Job drawing, mm, ordinate dimensions from the low corner. One solid piece. A direction names the side the tool comes from. Round coordinates to 2 decimals unless told otherwise and drop trailing zeros. Order: outer loops, then holes, each group sorted by start corner. A loop starts at its lowest first (then second) coordinate and runs counter-clockwise, first axis right, second up. Notation, with made-up numbers: (6.5, 57) -> (45.5, 57) arc R8 ccw to (45.5, 63) -> close; hole circle Ø8 at (40, -4.5). An arc over 180 degrees is marked (long way). Use CSV: the item, a comma, the result in double quotes.
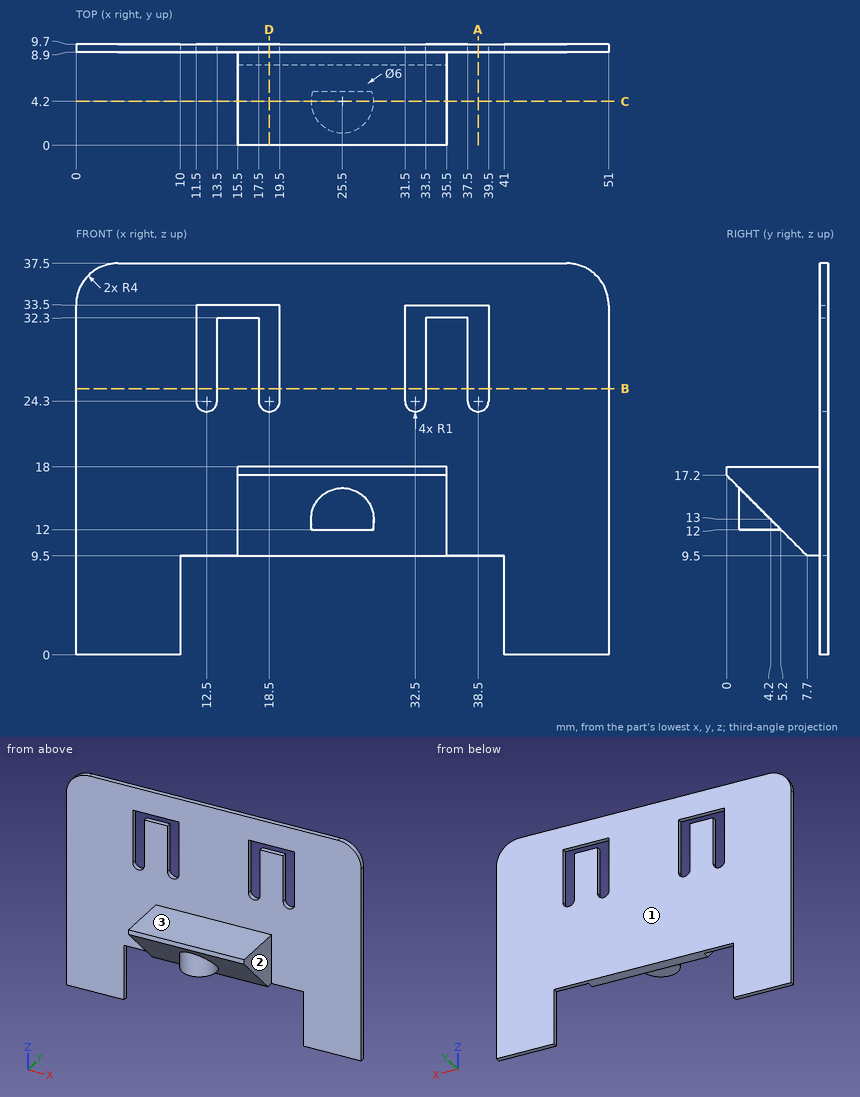
(1) Cut at D-D, the plane x = 18.5. Give the cut face in (y, z), then the cut area to 3 significant figures.
Reply:
outline,"(0, 17.2) -> (7.7, 9.5) -> (9.7, 9.5) -> (9.7, 23.3) -> (8.9, 23.3) -> (8.9, 18) -> (0, 18) -> close; (8.9, 33.5) -> (9.7, 33.5) -> (9.7, 37.5) -> (8.9, 37.5) -> close"
area,"60.2 mm2"
(2) Probe probe 1 along X at (y, z) = (9, 27); probe 2 along Y at (x, z) = (7.5, 16); probe 3 along X at (y, z) = (4.25, 17). List the from-to ranges inside material, lowest first. Write a range as [from, to].
Reply:
probe 1,"[0, 11.5], [13.5, 17.5], [19.5, 31.5], [33.5, 37.5], [39.5, 51]"
probe 2,"[8.9, 9.7]"
probe 3,"[15.5, 35.5]"
(3) Cut at B-B, the plane z = 25.5. Give the cut face in (x, y).
Reply:
outline,"(0, 8.9) -> (11.5, 8.9) -> (11.5, 9.7) -> (0, 9.7) -> close; (13.5, 8.9) -> (17.5, 8.9) -> (17.5, 9.7) -> (13.5, 9.7) -> close; (19.5, 8.9) -> (31.5, 8.9) -> (31.5, 9.7) -> (19.5, 9.7) -> close; (33.5, 8.9) -> (37.5, 8.9) -> (37.5, 9.7) -> (33.5, 9.7) -> close; (39.5, 8.9) -> (51, 8.9) -> (51, 9.7) -> (39.5, 9.7) -> close"
(4) Drop flat-ended pins along their axis: P1, Ø5, axis at x = 33.5, y = 5, coming from the -Z side; P2, Ø0.6, axis at x = 18.5, y = 8.5, coming from the -Z side; P3, Ø2.5, axis at y = 6, z = 15, coming from the +X side; P4, Ø1, axis at y = 1.5, z = 20, coming from the +X side. Give the stop position or say it passes through.
Reply:
P1,"z = 9.7"
P2,"z = 9.5"
P3,"x = 35.5"
P4,"through"
(5) Cut at C-C, the plane y = 4.2. Give the cut face in (x, z).
Reply:
outline,"(15.5, 13) -> (22.5, 13) -> (22.5, 12) -> (28.5, 12) -> (28.5, 13) -> (35.5, 13) -> (35.5, 18) -> (15.5, 18) -> close"
(6) Cut at A-A, the plane x = 38.5. Give the cut face in (y, z), then the cut area to 3 significant figures.
Reply:
outline,"(8.9, 9.5) -> (9.7, 9.5) -> (9.7, 23.3) -> (8.9, 23.3) -> close; (8.9, 33.5) -> (9.7, 33.5) -> (9.7, 37.5) -> (8.9, 37.5) -> close"
area,"14.2 mm2"
(7) Which spindle directions (+Z, -Z, +X, -X, +Y, -Y) get a long thin tool onto all of the face, cutting with end or side? Do the marked faces 1, 2 and 3. Say none if no direction does.
Reply:
face 1,"+Z, -Z, +X, -X, +Y"
face 2,"+Z, -Z, +X, -Y"
face 3,"+Z, +X, -X, -Y"
